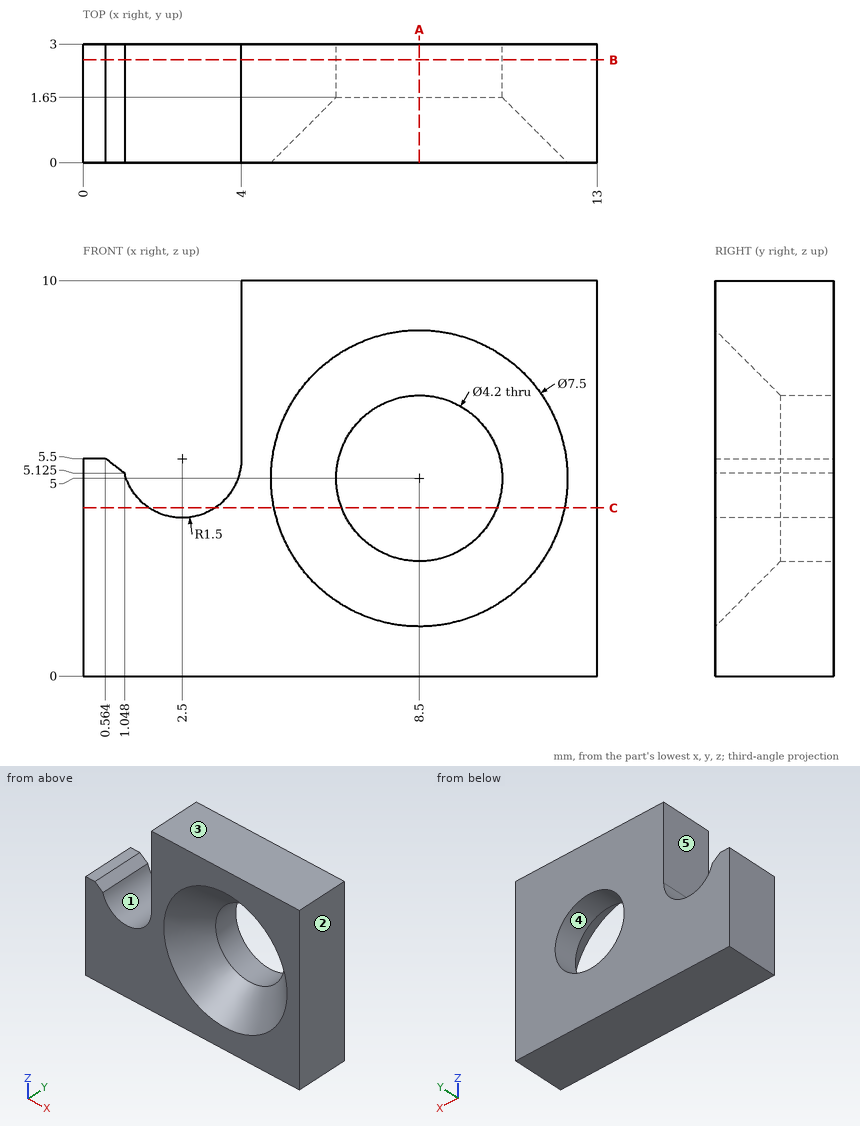
Answer from the drawing. Dimensions are ordinates in mm from the lowest x, y and z of the part. A direction names the side the tool comes from. Coordinates: 2 decimals unless noted, no trailing zeros. Loops run counter-clockwise (first coordinate to the right, second up) from the corner with the lowest first, then second, coordinate; pieces in that order, holes last. Notation, with made-up numbers: (7.25, -31.75) - (56.25, -31.75) arc R16 ccw to (56.25, -12.75) - close; hole circle Ø5 at (85, 25). An arc over 180 degrees is marked (long way). Use a Markdown table: item, result.
Item 1: Find section B-B, the plane y = 2.6. Determine the outline of the cut face in (x, z) (1 decimal).
Evaluation:
| item | result |
|---|---|
| outline | (0, 0) - (13, 0) - (13, 10) - (4, 10) - (4, 5.5) arc R1.5 cw to (1, 5.1) - (0.6, 5.5) - (0, 5.5) - close; hole circle Ø4.2 at (8.5, 5) |
Item 2: Find section A-A, the plane x = 8.5. Determine the outline of the cut face in (y, z).
Evaluation:
| item | result |
|---|---|
| outline | (0, 0) - (3, 0) - (3, 2.9) - (1.65, 2.9) - (0, 1.25) - close; (0, 8.75) - (1.65, 7.1) - (3, 7.1) - (3, 10) - (0, 10) - close |
Item 3: For the marked faces 4 and 5, determine the directions among +Z, -Z, +X, -X, +Y, -Y from which every point of the face is accessible in a straight line to the end or side of a thin tool.
Evaluation:
| item | result |
|---|---|
| face 4 | +Y, -Y |
| face 5 | +Z, -X, +Y, -Y |
Item 4: Given pin 1 Ø0.9 at (y, z) = (1.5, 8) entering from -X; pin 2 Ø0.5 at (x, y) = (0.5, 1.5) entering from +Z, each flat-ended and moving along its own axis, determine where each tip first touches the part or whether it passes through.
Evaluation:
| item | result |
|---|---|
| pin 1 | stops at x = 4 |
| pin 2 | stops at z = 5.5 |
Item 5: Find section C-C, the plane z = 4.25. State how many separate pieces and enclosed holes the cut face has, and give its area (3 significant figures).
Evaluation:
| item | result |
|---|---|
| separate pieces | 3 |
| enclosed holes | 0 |
| area | 19.4 mm2 |
Item 6: The mould has two halves that part along X. Classify the marked faces 1, 2 and 3: +X half, -X half, draft (parallel to the pull), parting line (faces both ways), or undercut.
Evaluation:
| item | result |
|---|---|
| face 1 | undercut |
| face 2 | +X half |
| face 3 | draft |
Item 7: Consider probe 1 along Z at (x, y) = (8.5, 2.55); probe 2 along X at (y, z) = (2.5, 5) (1 decimal); probe 3 along X at (y, z) = (0.8, 5.25) (1 decimal). Determine where each line is inside the solid, lowest interval first. Write a range as from..to.
Evaluation:
| item | result |
|---|---|
| probe 1 | z = 0..2.9, 7.1..10 |
| probe 2 | x = 0..1.1, 3.9..6.4, 10.6..13 |
| probe 3 | x = 0..0.9, 4..5.6, 11.4..13 |
